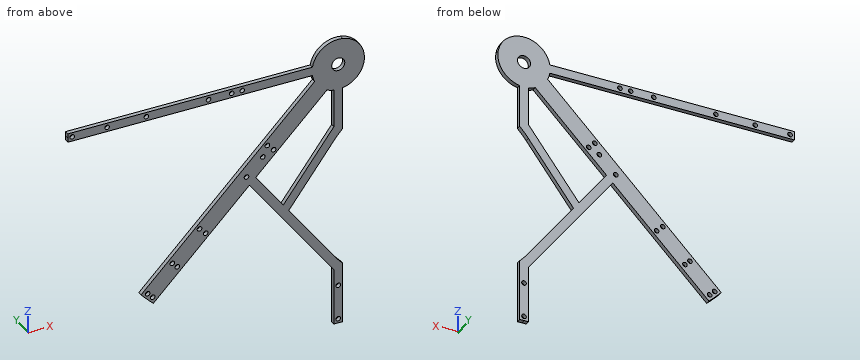
Autodesk Inventor part; units mm, degrees
ref_plane "YZ Plane" through (0, 0, 0) normal (1, 0, 0) x (0, 1, 0)
ref_plane "XZ Plane" through (0, 0, 0) normal (0, 1, 0) x (-1, 0, 0)
ref_plane "XY Plane" through (0, 0, 0) normal (0, 0, 1) x (1, 0, 0)
sketch "Sketch1" plane through (0, 0, 0) normal (0, 1, 0) x (-1, 0, 0)
  circle A0 centre (0, -139.7) radius 3.3782
  line L0 (6.35, -37.5671) -> (6.35, -393.6488)
  line L1 (-6.35, -37.5671) -> (-6.35, -393.7)
  circle A1 centre (193.0245, -202.0047) radius 3.3782
  circle A2 centre (202.0047, -193.0245) radius 3.3782
  line L2 (269.2628, -287.2233) -> (16.4197, -34.3803)
  line L3 (287.2233, -269.2628) -> (34.3803, -16.4197)
  circle A3 centre (94.1906, -103.1708) radius 3.3782
  circle A4 centre (103.1708, -94.1906) radius 3.3782
  circle A5 centre (139.7, 0) radius 3.3782
  line L4 (133.35, 0) -> (133.35, 6.35)
  line L5 (273.05, 6.35) -> (273.05, 0)
  line L6 (37.5671, -6.35) -> (393.6488, -6.35)
  line L7 (37.5671, 6.35) -> (393.7, 6.35)
  line L8 (146.05, 0) -> (146.05, 6.35)
  circle A6 centre (277.5195, -270.2276) radius 3.3782
  circle A7 centre (270.2276, -277.5195) radius 3.3782
  arc A8 (269.2628, -287.2233) -> (287.2233, -269.2628) centre (0, 0) ccw
  circle A9 centre (0, -387.35) radius 3.3782
  arc A10 (0, -393.7) -> (6.35, -393.6488) centre (0, 0) ccw
  line L9 (-6.35, -393.7) -> (0, -393.7)
  circle A11 centre (0, -279.4) radius 3.3782
  arc A12 (6.35, -37.5671) -> (16.4197, -34.3803) centre (0, 0) ccw
  arc A13 (34.3803, -16.4197) -> (37.5671, -6.35) centre (0, 0) ccw
  circle A14 centre (0, 0) radius 14.2875
  line L10 (38.1, 0) -> (38.1, 12.8556) construction
  arc A15 (-6.214, 37.5898) -> (-37.5898, 6.214) centre (0, 0) ccw
  arc A16 (37.5671, 6.35) -> (-6.35, -37.5671) centre (0, 0) ccw
  circle A17 centre (387.35, 0) radius 3.3782
  line L11 (393.7, 0) -> (393.7, 6.35)
  circle A18 centre (279.4, 0) radius 3.3782
  line L12 (285.75, 6.35) -> (285.75, 0)
  arc A19 (393.6488, -6.35) -> (393.7, 0) centre (0, 0) ccw
  line L13 (0, -285.75) -> (-6.35, -285.75)
  line L14 (-6.35, -273.05) -> (0, -273.05)
  circle A20 centre (0, -336.55) radius 3.3782
  circle A21 centre (241.5985, -234.3065) radius 3.3782
  circle A22 centre (234.3065, -241.5985) radius 3.3782
  circle A23 centre (336.55, 0) radius 3.3782
  dimension "d2" = 12.7
  dimension "d3" = 12.7
  dimension "d4" = 38.1
  dimension "d6" = 38.1
  dimension "d7" = 6.35
  dimension "d8" = 6.35
  dimension "d9" = 6.35
  dimension "d10" = 12.7
  dimension "d11" = 12.7
  dimension "d12" = 95.25
  dimension "d13" = 6.7564
  dimension "d14" = 6.7564
  dimension "d15" = 6.7564
  dimension "d16" = 6.35
  dimension "d17" = 6.7564
  dimension "d18" = 6.35
  dimension "d19" = 6.35
  dimension "d20" = 6.7564
  dimension "d21" = 6.7564
  dimension "d22" = 6.7564
  dimension "d23" = 6.35
  dimension "d24" = 6.7564
  dimension "d25" = 28.575
  dimension "d28" = 38.1
  dimension "d30" = 6.35
  dimension "d31" = 139.7
  dimension "d34" = 6.35
  dimension "d37" = 277.5195
  dimension "d38" = 270.2276
  dimension "d39" = 7.2919
  dimension "d40" = 7.2919
  dimension "d41" = 393.7
  dimension "d42" = 393.7
  dimension "d43" = 6.35
  dimension "d44" = 12.7
  dimension "d45" = 6.7564
  dimension "d46" = 6.35
  dimension "d47" = 6.7564
  dimension "d48" = 6.7564
  dimension "d49" = 393.7
  dimension "d50" = 6.35
  dimension "d51" = 6.7564
  dimension "d52" = 6.35
  dimension "d54" = 6.7564
  dimension "d55" = 6.7564
  dimension "d56" = 6.7564
  dimension "d57" = 50.8
  dimension "d58" = 50.8
  dimension "d59" = 50.8
  dimension "d60" = 7.5438
  dimension "d61" = 7.5438
  dimension "d62" = 7.5438
  dimension "d63" = 7.5438
  dimension "d64" = 50.8
extrude "Extrusion1" add sketch "Sketch1" along normal blind 6.35
sketch "Sketch7" plane through (0, 6.35, 0) normal (0, 1, 0) x (1, 0, 0)
  circle A0 centre (0, 0) radius 14.2875
  circle A1 centre (0, 0) radius 9.5
  dimension "d99" = 19
extrude "Extrusion6" add sketch "Sketch7" against normal blind 6.35
sketch "Sketch9" plane through (0, 6.35, 0) normal (0, 1, 0) x (1, 0, 0)
  circle A0 centre (0, 139.7) radius 3.3782
  circle A1 centre (0, 279.4) radius 3.3782
  arc A2 (104.14, 347.9822) -> (104.1415, 56.1583) centre (110.49, 202.0703) ccw
  circle A3 centre (110.49, 202.0703) radius 146.05
  dimension "d102" = 0
  dimension "d103" = 0
  dimension "d104" = 0
extrude "Extrusion7" cut sketch "Sketch9" against normal blind 25.4
sketch "Sketch10" plane through (0, 6.35, 0) normal (0, 1, 0) x (1, 0, 0)
  arc A0 (6.35, 304.4688) -> (-6.35, 289.7003) centre (110.49, 202.0703) ccw
  line L0 (-6.35, 393.6488) -> (-6.35, 289.7003)
  arc A1 (-6.35, 114.4403) -> (6.35, 99.6717) centre (110.49, 202.0703) ccw
  line L1 (-6.35, 114.4403) -> (-6.35, 37.5671)
  arc A2 (-6.35, 37.5671) -> (-16.4197, 34.3803) centre (0, 0) ccw
  line L2 (-16.4197, 34.3803) -> (-269.2628, 287.2233)
  arc A3 (-269.2628, 287.2233) -> (-287.2233, 269.2628) centre (0, 0) ccw
  line L3 (-287.2233, 269.2628) -> (-34.3803, 16.4197)
  arc A4 (-34.3803, 16.4197) -> (-37.5671, 6.35) centre (0, 0) ccw
  line L4 (-37.5671, 6.35) -> (-393.6488, 6.35)
  arc A5 (-393.6488, 6.35) -> (-393.7, 0) centre (0, 0) ccw
  line L5 (-393.7, 0) -> (-393.7, -6.35)
  line L6 (-393.7, -6.35) -> (-37.5671, -6.35)
  arc A6 (-37.5671, -6.35) -> (6.35, 37.5671) centre (0, 0) ccw
  line L7 (6.35, 37.5671) -> (6.35, 99.6717)
  circle A7 centre (0, 0) radius 9.5
  circle A8 centre (-270.2276, 277.5195) radius 3.3782
  circle A9 centre (-277.5195, 270.2276) radius 3.3782
  circle A10 centre (-234.3065, 241.5985) radius 3.3782
  circle A11 centre (-241.5985, 234.3065) radius 3.3782
  circle A12 centre (-387.35, 0) radius 3.3782
  circle A13 centre (-336.55, 0) radius 3.3782
  circle A14 centre (-139.7, 0) radius 3.3782
  circle A15 centre (-279.4, 0) radius 3.3782
  circle A16 centre (-94.1906, 103.1708) radius 3.3782
  circle A17 centre (-103.1708, 94.1906) radius 3.3782
  circle A18 centre (-193.0245, 202.0047) radius 3.3782
  circle A19 centre (-202.0047, 193.0245) radius 3.3782
  line L8 (-6.35, 114.4403) -> (-72.0725, 202.0703)
  line L9 (-6.35, 310.8669) -> (-129.1599, 147.1204)
  line L10 (-80.01, 191.4869) -> (-6.35, 93.2736)
  line L11 (-6.35, 289.7003) -> (-72.0725, 202.0703)
  line L12 (-80.01, 191.4869) -> (-120.0885, 138.049)
extrude "Extrusion8" add sketch "Sketch10" against normal blind 6.35 contours L0 L11 L8 L1 L10 L12 L2 L9
sketch "Sketch11" plane through (0, 6.35, 0) normal (0, 1, 0) x (1, 0, 0)
  circle A0 centre (-109.7506, 109.7506) radius 3.3782
  circle A1 centre (-133.5483, 133.5483) radius 3.3782
  circle A2 centre (-188.8658, 0) radius 3.3782
  circle A3 centre (-155.2108, 0) radius 3.3782
extrude "Extrusion9" cut sketch "Sketch11" against normal blind 25.4
equation "\"d60\" = d63"
equation "\"d61\" = d62"
properties part number "Bearing Mount Top" material "Aluminum 6061"
For this review, take the finished solid that the model builds, in its own axes (mm). Round coordinates to 2 decimals unless told otherwise and drop trailing zeros. Write each loop counter-clockwise with the first axis right and the second up, starting at its lowest first coordinate (ties: lowest second). Pieces come first, ordered by that corner, then holes. Notation, with made-up numbers: M -35.5,-35.5 L -10.5,-35.5 A14 ccw -10.5,-22.5 Z; hole C 50.5,2.25 d7. An arc over 180 degrees is marked long. One line per item, written item: value. Start each with the question number.
(1) Wall thickness on line 1 (Z direction, x = -336.55, y = 4.75); line 2 (Z direction, x = -25.5, y = 1.5): over which ranges is each line inside the solid? List them lowest first.
(2) We need section B-B (x = -297). Give the boundary of the cut face in (y, z).
(3) We need section A-A (z = -45). Give the boundary of the cut face in (x, y).
(4) Insertion check: pin 1 (1.9 mm diameter, centred on x = -191.5, y = 4.5, fed in from +Z); pin 2 (6 mm diameter, centred on x = -109.75, z = -109.75, fed in from +Y); pin 3 (9 mm diameter, centred on x = -277.52, z = -270.23, fed in from +Y); pin 4 (2 mm diameter, centred on y = 5, z = -41, fed in from -X). Each pin has a flat end and moves straight along its axis. Give the tip position at first contact, or say it passes through.
(5) We need section D-D (z = -316). Give the boundary of the cut face in (x, y).
(6) We need section C-C (y = 4.25). Count the separate pieces of the cut face and the enclosed holes in it, and give its area (3 significant figures).
Result:
1. line 1: -6.35 to -3.38, 3.38 to 6.35
1. line 2: -285.33 to -264.17, -139.97 to -118.81, -43.46 to 28.31
2. outline: M 0,-6.35 L 6.35,-6.35 L 6.35,6.35 L 0,6.35 Z
3. outline: M -62.96,0 L -27.04,0 L -27.04,6.35 L -62.96,6.35 Z; M -6.35,0 L 6.35,0 L 6.35,6.35 L -6.35,6.35 Z
4. pin 1: z = 6.35
4. pin 2: through
4. pin 3: y = 6.35
4. pin 4: x = -59.96
5. outline: M -6.35,0 L 6.35,0 L 6.35,6.35 L -6.35,6.35 Z
6. separate pieces: 1
6. enclosed holes: 20
6. area: 23,300 mm²
